Input: part model. Units: mm. Frame: model coordinates. Face numbers are marked on the shaded views. A direction names the side the tool comes from. Give positions to 0.01 mm unless a question says otherwise; leave off trailing zeros. Write each loop counter-clockwise with the first axis right and the second up, starting at its lowest first coordinate (ties: lowest second). Pieces come first, ordered by that corner, then holes. Notation, with made-up numbers: (-11.75, 47.5) - (44.25, 47.5) arc R12 ccw to (44.25, 59.5) - close; hole circle Ø10 at (48.25, 21). An arc over 180 degrees is marked (long way). Use a Markdown table: item, result. Add a question column.
1. Section query D-D, the plane x = -5. Return loops of the section in (y, z).
2. Section query B-B, the plane x = 23. Count the separate pieces of the cut face and the enclosed holes in it, plus the area to 3 significant figures.
3. Material intervals for probe 1 along Z at (x, y) = (-4.5, 0); probe 2 along Z at (x, y) = (25.5, -23.5); probe 3 along Y at (x, z) = (20.5, 4), sorted ascending.
4. Pin query (flat end, axial travel): pin 1 (8 mm diameter, centred on x = -5, z = -49, fed in from +Y); pin 2 (12 mm diameter, centred on x = -5.5, z = -7, fed in from +Y); pin 3 (3.5 mm diameter, centred on x = -8.5, y = 37, fed in from +Z); pin 4 (6 mm diameter, centred on x = -5, y = 37, fed in from -Z). Return the tip coordinate at first contact, or that it passes through.
5. Section query C-C, the plane z = 0. Return loops of the section in (x, y), plus the area to 3 significant figures.
6. Section query A-A, the plane y = 0. Return loops of the section in (x, z), plus the area to 4 significant figures.
7. Mould query, pull axis Y, two halves, no side actions, for the marked faces 4, 5 and 6. Classes: released by +Y, released by -Y, zero draft, split by the parting line, or undercut.
8. Set-up query: the marked faces 1, 2 and 3. Return all of +Z, -Z, +X, -X, +Y, -Y with unobstructed straight access to the full face (end or side cutting, diameter ignored); none if empty.
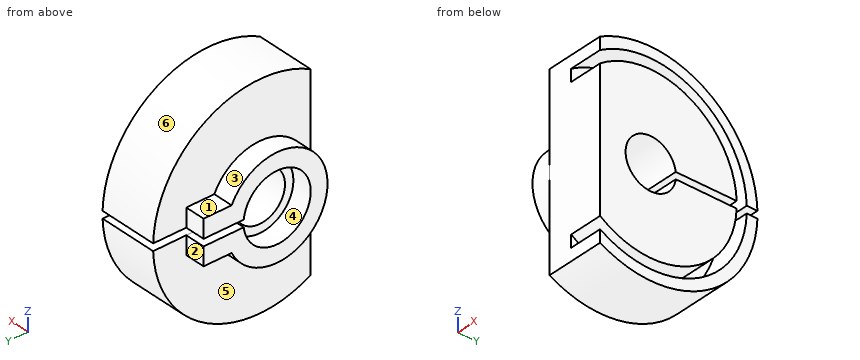
```python
from build123d import *

# Parameters (mm, degrees)
SALIENTE_EXTRUIR1_DEPTH = 35
SALIENTE_EXTRUIR2_DEPTH = 12
CROQUIS2_R              = 57.15
CROQUIS2_R_2            = 51.15
CORTAR_EXTRUIR2_DEPTH   = 20
CORTAR_EXTRUIR3_REACH   = 98.382
CROQUIS4_W              = 151.714378115
CROQUIS4_H              = 39.157803324


with BuildPart() as part:
    # Croquis1 → Saliente-Extruir1 (new body)
    with BuildSketch(Plane(origin=(0, 0, 0), x_dir=(0, 0, -1), z_dir=(1, 0, 0))):
        with BuildLine():
            Line((-2, 14.866068747), (-2, 63.468496122))
            ThreePointArc((-2, 63.468496122), (-0.098669817, -63.499923341), (2.197231834, 63.461974223))
            Line((2.197231834, 63.461974223), (2, 14.866068747))
            ThreePointArc((2, 14.866068747), (0, -15), (-2, 14.866068747))
        make_face()
    extrude(amount=SALIENTE_EXTRUIR1_DEPTH)

    # Croquis3 → Saliente-Extruir2 (add)
    with BuildSketch(Plane.ZY):
        with BuildLine():
            Line((-2.1172783, 19.887612541), (-2.1172783, 43.76224174))
            Line((-2.1172783, 43.76224174), (-12.9131853, 43.76224174))
            Line((-12.9131853, 43.76224174), (-12.9131853, 27.07858278))
            ThreePointArc((-12.9131853, 27.07858278), (0, -30), (12.9131853, 27.07858278))
            Line((12.9131853, 27.07858278), (12.9131853, 43.76224174))
            Line((12.9131853, 43.76224174), (2, 43.76224174))
            Line((2, 43.76224174), (2, 19.899748742))
            ThreePointArc((2, 19.899748742), (0.058952284, -19.999913116), (-2.1172783, 19.887612541))
        make_face()
    extrude(amount=SALIENTE_EXTRUIR2_DEPTH)

    # Croquis2 → Cortar-Extruir2 (cut)
    with BuildSketch(Plane.ZY.offset(-35)):
        Circle(CROQUIS2_R)
        Circle(CROQUIS2_R_2, mode=Mode.SUBTRACT)
    extrude(amount=CORTAR_EXTRUIR2_DEPTH, mode=Mode.SUBTRACT)

    # Croquis4 → Cortar-Extruir3 (cut, up to next)
    with BuildSketch(Plane.ZY, mode=Mode.PRIVATE) as cortar_extruir3_sk1:
        with Locations((-1.340233023, -49.726897526)):
            Rectangle(CROQUIS4_W, CROQUIS4_H)
    cortar_extruir3_tool1 = extrude(cortar_extruir3_sk1.sketch, amount=-CORTAR_EXTRUIR3_REACH, mode=Mode.PRIVATE) & part.part
    add(cortar_extruir3_tool1.solids().sort_by_distance((0, -49.726898, -1.340233))[0], mode=Mode.SUBTRACT)


solid = part.part
```
Result sheet:
| question | item | result |
|---|---|---|
| 1 | outline | (19.89, -2.12) arc R20 cw (long way) to (19.9, 2) - (43.76, 2) - (43.76, 12.91) - (27.08, 12.91) arc R30 ccw (long way) to (27.08, -12.91) - (43.76, -12.91) - (43.76, -2.12) - close |
| 2 | separate pieces | 3 |
| 2 | enclosed holes | 0 |
| 2 | area | 7,730 mm² |
| 3 | probe 1 | z = -30 to -20, 20 to 30 |
| 3 | probe 2 | z = -58.99 to -52.09, -45.43 to 45.43, 52.09 to 58.99 |
| 3 | probe 3 | y = -30.15 to -14.46, 14.46 to 50.99, 57.01 to 63.37 |
| 4 | pin 1 | passes through |
| 4 | pin 2 | stops at y = 63.33 |
| 4 | pin 3 | stops at z = 12.91 |
| 4 | pin 4 | stops at z = -12.91 |
| 5 | outline | (-12, -30) - (0, -30) - (0, -30.15) - (35, -30.15) - (35, -15) - (0, -15) - (0, -20) - (-12, -20) - close |
| 5 | area | 650 mm² |
| 6 | outline | (-12, -30) - (0, -30) - (0, -63.5) - (35, -63.5) - (35, -57.15) - (15, -57.15) - (15, -51.15) - (35, -51.15) - (35, -15) - (0, -15) - (0, -20) - (-12, -20) - close; (-12, 20) - (0, 20) - (0, 15) - (35, 15) - (35, 51.15) - (15, 51.15) - (15, 57.15) - (35, 57.15) - (35, 63.5) - (0, 63.5) - (0, 30) - (-12, 30) - close |
| 6 | area | 3,395 mm² |
| 7 | face 4 | undercut |
| 7 | face 5 | zero draft |
| 7 | face 6 | split by the parting line |
| 8 | face 1 | +Z, -X, +Y |
| 8 | face 2 | +Z, -Z, -X, +Y |
| 8 | face 3 | -X |
